Part model, mm, in its own coordinate system. Face numbers are marked on the shaded views. A direction names the side the tool comes from. Coordinates: 2 decimals unless noted, no trailing zeros. Order: outer loops, then holes, each group sorted by start corner. A loop starts at its lowest first (then second) coordinate and runs counter-clockwise, first axis right, second up.
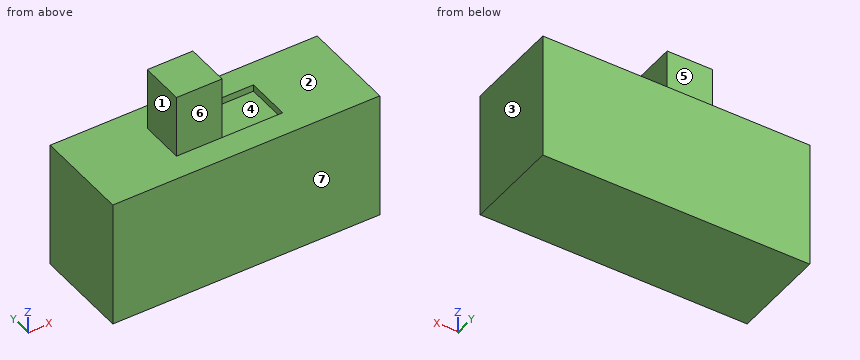
```python
from build123d import *

# Parameters (mm, degrees)
SKETCH1_W           = 11.72
SKETCH1_H           = 5.6
BOSS_EXTRUDE1_DEPTH = 4.2
SKETCH2_W           = 2
SKETCH2_H           = 1.96
BOSS_EXTRUDE2_DEPTH = 2.76
SKETCH2_3_W         = 2.66
SKETCH2_3_H         = 1.96
CUT_EXTRUDE1_DEPTH  = 0.3


with BuildPart() as part:
    # Sketch1 → Boss-Extrude1 (new body)
    with BuildSketch(Plane(origin=(0, 0, 0), x_dir=(1, 0, 0), z_dir=(0, 1, 0))):
        Rectangle(SKETCH1_W, SKETCH1_H)
    extrude(amount=BOSS_EXTRUDE1_DEPTH)

    # Sketch2 → Boss-Extrude2 (add)
    with BuildSketch(Plane.XY.offset(2.8)):
        with Locations((-1.33, 2.1)):
            Rectangle(SKETCH2_W, SKETCH2_H)
    extrude(amount=BOSS_EXTRUDE2_DEPTH)

    # Sketch2<3> → Cut-Extrude1 (cut)
    with BuildSketch(Plane.XY.offset(2.8)):
        with Locations((1, 2.1)):
            Rectangle(SKETCH2_3_W, SKETCH2_3_H)
    extrude(amount=-CUT_EXTRUDE1_DEPTH, mode=Mode.SUBTRACT)


solid = part.part
```
(1) Slice it at C-C, the plane z = 5. Give the cut face in (x, y), then the cut area to 3 significant figures.
(2) Drop flat-ended pins along their axis: pin 1 (2 mm diameter, centred on x = -1.5, z = 4, fed in from -Y); pin 2 (2 mm diameter, centred on y = 2, z = 4.5, fed in from -X); pin 3 (1 mm diameter, centred on x = 2.5, y = 1, fed in from +Z). Give the stop position or say it passes through.
(3) Slice it at A-A, the plane x = 0.25. Give the cut face in (y, z), then the cut area to 3 significant figures.
(4) Probe line 1 (X direction, y = 1.5, z = 2.75); line 2 (Z direction, x = -1.25, y = 3.25); line 3 (X direction, y = 1.6, z = 4.75). List the from-to ranges inside material, lowest first.
(5) Slice it at B-B, the plane y = 1.6. Give the cut face in (x, z), then the cut area to 3 significant figures.
(6) Slice it at D-D, the plane x = 4.75. Give the cut face in (y, z), then the cut area to 3 significant figures.
(7) Tool access for the marked faces 5, 6 and 7: list every direction of +Z, -Z, +X, -X, +Y, -Y with a clear straight run to the whole face (end or side of a thin tool).
(8) Pull direction X, two halves, no side cores. Call the marked faces 1, 2, 3 and 4: +X half, -X half, draft (parallel to the pull), parting line (faces both ways), or undercut.
Here are the results:
1. outline: (-2.33, 1.12) - (-0.33, 1.12) - (-0.33, 3.08) - (-2.33, 3.08) - close
1. area: 3.92 mm2
2. pin 1: stops at y = 1.12
2. pin 2: stops at x = -2.33
2. pin 3: stops at z = 2.8
3. outline: (0, -2.8) - (4.2, -2.8) - (4.2, 2.8) - (3.08, 2.8) - (3.08, 2.5) - (1.12, 2.5) - (1.12, 2.8) - (0, 2.8) - close
3. area: 22.9 mm2
4. line 1: x = -5.86 to -0.33, 2.33 to 5.86
4. line 2: z = -2.8 to 2.8
4. line 3: x = -2.33 to -0.33
5. outline: (-5.86, -2.8) - (5.86, -2.8) - (5.86, 2.8) - (2.33, 2.8) - (2.33, 2.5) - (-0.33, 2.5) - (-0.33, 5.56) - (-2.33, 5.56) - (-2.33, 2.8) - (-5.86, 2.8) - close
5. area: 70.4 mm2
6. outline: (0, -2.8) - (4.2, -2.8) - (4.2, 2.8) - (0, 2.8) - close
6. area: 23.5 mm2
7. face 5: +Z, +X, -X, +Y
7. face 6: +Z, +X, -X, -Y
7. face 7: +Z, -Z, +X, -X, -Y
8. face 1: -X half
8. face 2: draft
8. face 3: +X half
8. face 4: undercut
